from build123d import *

# Parameters (mm, degrees)
SKETCH_W        = 31.75
SKETCH_H        = 31.75
PAD_DEPTH       = 15.875
SKETCH001_R     = 11
POCKET_DEPTH    = 7
SKETCH002_R     = 8
POCKET001_DEPTH = 34.926
SKETCH003_R     = 1.25
HOLE_DEPTH      = 31.751
SKETCH004_R     = 1.25
HOLE001_DEPTH   = 20
HOLE001_TIPS_R  = 1.25


with BuildPart() as part:
    # Sketch → Pad (new body, symmetric)
    with BuildSketch(Plane.XY):
        Rectangle(SKETCH_W, SKETCH_H)
    extrude(amount=PAD_DEPTH, both=True)

    # Sketch001 (on Face6 of Pad) → Pocket (cut)
    with BuildSketch(Plane.XY.offset(15.875)):
        Circle(SKETCH001_R)
    extrude(amount=-POCKET_DEPTH, mode=Mode.SUBTRACT)

    # Sketch002 → Pocket001 (cut, through all)
    with BuildSketch(Plane.XY.offset(19.05)):
        Circle(SKETCH002_R)
    extrude(amount=-POCKET001_DEPTH, mode=Mode.SUBTRACT)

    # Sketch003 (on Face6 of Pocket001) → Hole (cut, through all)
    with BuildSketch(Plane.YZ.offset(15.875)):
        with Locations((-12.5, 12.5)):
            Circle(SKETCH003_R)
        with Locations((12.5, 12.5)):
            Circle(SKETCH003_R)
        with Locations((9.5, -12.5)):
            Circle(SKETCH003_R)
        with Locations((-9.5, -12.5)):
            Circle(SKETCH003_R)
    extrude(amount=-HOLE_DEPTH, mode=Mode.SUBTRACT)

    # Sketch004 (on Face4 of Pocket001) → Hole001 (cut)
    with BuildSketch(Plane(origin=(0, 0, -15.875), x_dir=(1, 0, 0), z_dir=(0, 0, -1))):
        with Locations((-12.5, 12.5)):
            Circle(SKETCH004_R)
        with Locations((12.5, 12.5)):
            Circle(SKETCH004_R)
        with Locations((12.5, -12.5)):
            Circle(SKETCH004_R)
        with Locations((-12.5, -12.5)):
            Circle(SKETCH004_R)
    extrude(amount=-HOLE001_DEPTH, mode=Mode.SUBTRACT)

    # Hole001 tips → Hole001 tip 1 section 0
    with BuildSketch(Plane(origin=(0, 0, 4.125), x_dir=(1, 0, 0), z_dir=(0, 0, -1)), mode=Mode.PRIVATE) as hole001_tip_1_s0:
        with Locations((-12.5, 12.5)):
            Circle(HOLE001_TIPS_R)
    loft([hole001_tip_1_s0.sketch, Vertex(-12.5, -12.5, 4.876076)], mode=Mode.SUBTRACT)

    # Hole001 tips → Hole001 tip 2 section 0
    with BuildSketch(Plane(origin=(0, 0, 4.125), x_dir=(1, 0, 0), z_dir=(0, 0, -1)), mode=Mode.PRIVATE) as hole001_tip_2_s0:
        with Locations((12.5, 12.5)):
            Circle(HOLE001_TIPS_R)
    loft([hole001_tip_2_s0.sketch, Vertex(12.5, -12.5, 4.876076)], mode=Mode.SUBTRACT)

    # Hole001 tips → Hole001 tip 3 section 0
    with BuildSketch(Plane(origin=(0, 0, 4.125), x_dir=(1, 0, 0), z_dir=(0, 0, -1)), mode=Mode.PRIVATE) as hole001_tip_3_s0:
        with Locations((12.5, -12.5)):
            Circle(HOLE001_TIPS_R)
    loft([hole001_tip_3_s0.sketch, Vertex(12.5, 12.5, 4.876076)], mode=Mode.SUBTRACT)

    # Hole001 tips → Hole001 tip 4 section 0
    with BuildSketch(Plane(origin=(0, 0, 4.125), x_dir=(1, 0, 0), z_dir=(0, 0, -1)), mode=Mode.PRIVATE) as hole001_tip_4_s0:
        with Locations((-12.5, -12.5)):
            Circle(HOLE001_TIPS_R)
    loft([hole001_tip_4_s0.sketch, Vertex(-12.5, 12.5, 4.876076)], mode=Mode.SUBTRACT)


solid = part.part
Geometry check sheet. Reference: the model listing, model coordinates, mm. A direction names the side the tool comes from. Give positions to 0.01 mm unless a question says otherwise; leave off trailing zeros. Order: outer loops, then holes, each group sorted by start corner. A loop starts at its lowest first (then second) coordinate and runs counter-clockwise, first axis right, second up. Notation, with made-up numbers: (28, 84) - (44, 84) arc R18 ccw to (44, 105) - close; hole circle Ø6 at (-26, -29). An arc over 180 degrees is marked (long way). Use one line per item in the form item = value.
1) Sectioned sample at C-C (z = 12.5). Record the boundary of the cut face in (x, y) (3 decimals), and give its area (3 significant figures).
Working result:
outline = (-15.875, -15.875) - (15.875, -15.875) - (15.875, -13.75) - (-15.875, -13.75) - close; (-15.875, -11.25) - (15.875, -11.25) - (15.875, 11.25) - (-15.875, 11.25) - close; (-15.875, 13.75) - (15.875, 13.75) - (15.875, 15.875) - (-15.875, 15.875) - close; hole circle Ø22 at (0, 0)
area = 469 mm^2
2) Draft check along Y on faces 1 (the face through (15.875, 0, 0)), 2 (the face through (0, 15.875, 0)), 3 (the face through (-12.658, -12.379, 4.756)). Enter one of: released by +Y, released by -Y, zero draft, split by the parting line, or undercut.
Working result:
face_1 = zero draft
face_2 = released by +Y
face_3 = undercut
3) Depth check by flat-ended pin: pin 1 Ø1 at (x, y) = (-5.5, -3) entering from -Z; pin 2 Ø2 at (x, y) = (-12.5, 12.5) entering from -Z. Enter the tip coordinate at first touch or a pass-through.
Working result:
pin_1 = through
pin_2 = 4.28
4) Sectioned sample at B-B (x = 6). Count the separate pieces of the cut face and the enclosed holes in it, and give its area (3 significant figures).
Working result:
separate_pieces = 2
enclosed_holes = 4
area = 597 mm^2
5) Access from +Z, -Z, +X, -X, +Y, -Y to the whole of each face (thin tool, end or side, straight path). Record for faces 4 (the face through (-2.38, -10.74, 12.42)), 5 (the face through (12.34, 11.26, -6.02)), 6 (the face through (0.222, -10.421, -11.655)).
Working result:
face_4 = +Z
face_5 = -Z
face_6 = +X, -X
6) Sectioned sample at D-D (z = 1). Record the boundary of the cut face in (x, y) (3 decimals).
Working result:
outline = (-15.875, -15.875) - (15.875, -15.875) - (15.875, 15.875) - (-15.875, 15.875) - close; hole circle Ø2.5 at (-12.5, -12.5); hole circle Ø2.5 at (-12.5, 12.5); hole circle Ø16 at (0, 0); hole circle Ø2.5 at (12.5, -12.5); hole circle Ø2.5 at (12.5, 12.5)
7) Material ranges on probe 1 along Y at (x, z) = (-12.5, -6.5) (3 decimals); probe 2 along Y at (x, z) = (-12, -5) (3 decimals); probe 3 along Y at (x, z) = (0, -8.75) (3 decimals), recorded low to high. Write a range as from..to.
Working result:
probe_1 = -15.875..-13.75, -11.25..11.25, 13.75..15.875
probe_2 = -15.875..-13.646, -11.354..11.354, 13.646..15.875
probe_3 = -15.875..-8, 8..15.875
8) Sectioned sample at A-A (z = -12.5). Record the boundary of the cut face in (x, y) (3 decimals), and give its area (3 significant figures).
Working result:
outline = (-15.875, -15.875) - (15.875, -15.875) - (15.875, -10.75) - (-15.875, -10.75) - close; (-15.875, -8.25) - (15.875, -8.25) - (15.875, 8.25) - (-15.875, 8.25) - close; (-15.875, 10.75) - (15.875, 10.75) - (15.875, 15.875) - (-15.875, 15.875) - close; hole circle Ø2.5 at (-12.5, -12.5); hole circle Ø2.5 at (-12.5, 12.5); hole circle Ø16 at (0, 0); hole circle Ø2.5 at (12.5, -12.5); hole circle Ø2.5 at (12.5, 12.5)
area = 629 mm^2
